Here's how the part is built. I have some questions about the finished solid (model axes, mm). Coordinates: 2 decimals unless noted, no trailing zeros. Loops run counter-clockwise (first coordinate to the right, second up) from the corner with the lowest first, then second, coordinate; pieces in that order, holes last. Notation, with made-up numbers: (31.25, 6.5) -> (60.25, 6.5) arc R24 cw to (60.25, 21.5) -> close; hole circle Ø10 at (34.5, -20). An arc over 180 degrees is marked (long way). Answer as a JSON object with one key per item and string values. Group by question number.
1) I want a section at B-B (y = 84). Write out the boundary of the cut face in (x, z).
2) If we mould it in two halves opening along Z, with no side actions, what happens to faces 1 (the flat face through (-26, 38, -12.192)), 2 (the cylindrical face through (-25.234, 101.806, 22.835)), 3 (the flat face through (-42.362, 51, 11))? For each: +Z half, -Z half, draft (parallel to the pull), parting line (faces both ways), or undercut.
3) I want a section at C-C (z = 31). Write out the boundary of the cut face in (x, y), then the cut area to 3 significant figures.
4) I need wall thicknesses on probe 1 along Z at (x, y) = (-33.5, 29); probe 2 along Z at (x, y) = (-24, 14). Which ranges of each line are inside material? Lowest first, please. Write a range as [from, to].
5) I'm going to push flat-ended pins straight in: pin 1 (2 mm diameter, centred on x = -21, z = 31.5, fed in from +Y); pin 2 (1 mm diameter, centred on x = -37, y = 13, fed in from +Z). Where does each tip first touch, or does it pass through?
6) I want a section at A-A (x = -21). Write out the boundary of the cut face in (y, z), then the cut area to 3 significant figures.
```python
from build123d import *

# Parameters (mm, degrees)
F0_W     = 33.782
F0_H     = 133.35
F1_ANGLE = 20
F2_DEPTH = 12.192


with BuildPart() as f1:
    # F0 (on Top) → F1 (revolve)
    with BuildSketch(Plane.XY):
        with Locations((-25.47081, 37.101181)):
            Rectangle(F0_W, F0_H)
    revolve(axis=Axis((-25.47081, -29.573819, 0), (1, 0, 0)), revolution_arc=F1_ANGLE)

    # F0 (on Top) → F2 (join)
    with BuildSketch(Plane.XY):
        with Locations((-25.47081, 37.101181)):
            Rectangle(F0_W, F0_H)
    extrude(amount=-F2_DEPTH)


solid = f1.part
```
Determined:
{
 "1": {"outline": "(-42.36, -12.19) -> (-8.58, -12.19) -> (-8.58, 41.34) -> (-42.36, 41.34) -> close"},
 "2": {"face 1": "-Z half", "face 2": "+Z half", "face 3": "draft"},
 "3": {"outline": "(-42.36, 55.6) -> (-8.58, 55.6) -> (-8.58, 100.12) -> (-42.36, 100.12) -> close", "area": "1,500 mm^2"},
 "4": {"probe 1": "[-12.19, 21.32]", "probe 2": "[-12.19, 15.86]"},
 "5": {"pin 1": "y = 100.24", "pin 2": "z = 15.68"},
 "6": {"outline": "(-29.57, -12.19) -> (103.78, -12.19) -> (103.78, 0) arc R133.35 ccw to (95.73, 45.61) -> (-29.57, 0) -> close", "area": "4,730 mm^2"}
}
